Could you check a few things on this drawing? It's one solid part, dimensions in mm from its lowest x, y, z. A direction names the side the tool comes from. Round coordinates to 2 decimals unless told otherwise and drop trailing zeros. Order: outer loops, then holes, each group sorted by start corner. A loop starts at its lowest first (then second) coordinate and runs counter-clockwise, first axis right, second up. Notation, with made-up numbers: M -21,58.25 L 37,58.25 A22 cw 37,83.25 Z; hole C -2.75,-29.5 d9. An arc over 180 degrees is marked long. Answer as a JSON object with one key per item and string values. Group by question number.
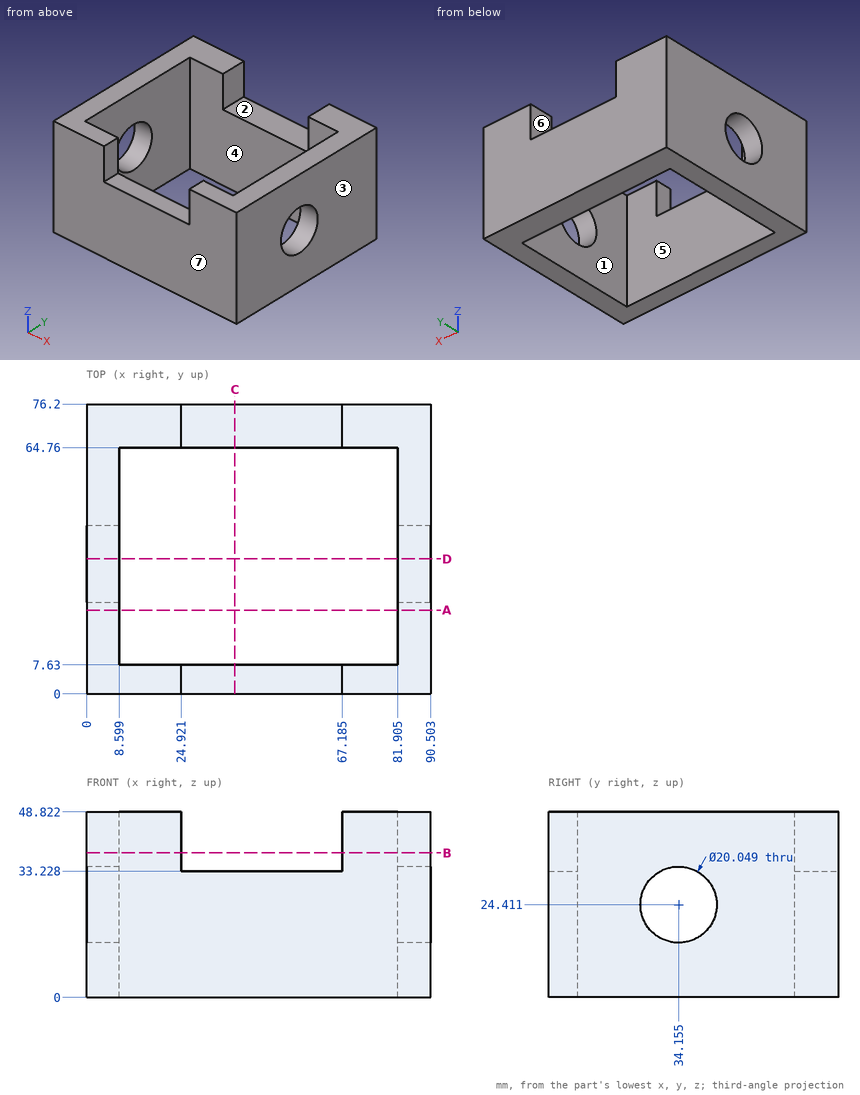
1) If we section it at B-B on z = 38: Write out the boundary of the cut face in (x, y) (1 decimal), plus the area to 3 significant figures.
2) If we section it at C-C on x = 39: Write out the boundary of the cut face in (y, z), plus the area to 3 significant figures.
3) If we section it at A-A on y = 22: Write out the boundary of the cut face in (x, z) (1 decimal).
4) Which directions (+Z, -Z, +X, -X, +Y, -Y) give clear straight access to the entire face, cutting with the end or side of a thin tool? Please do the marked faces 1, 2 and 3.
5) We'd pull the mould along Y, two halves only. Please class the marked faces 4, 5, 6 and 7: +Y half, -Y half, draft (parallel to the pull), parting line (faces both ways), or undercut.
6) If we section it at D-D on y = 35.5: Write out the boundary of the cut face in (x, z) (1 decimal).
7) For pin 1 (4 mm diameter, centred on x = 41.5, y = 5.5, fed in from +Z), with a flat end and sliding along its axis, tell me the tip position at first contact or that it passes through.
8) I need wall thicknesses on line 1 along Y through (x, z) = (38.5, 11); line 2 along X through (y, z) = (32, 35) (1 decimal); line 3 along Z through (x, y) = (44.5, 68). Which ranges of each line are inside material? Lowest first, please.
Findings:
{
 "1": {"outline": "M 0,0 L 24.9,0 L 24.9,7.6 L 8.6,7.6 L 8.6,64.8 L 24.9,64.8 L 24.9,76.2 L 0,76.2 Z; M 67.2,0 L 90.5,0 L 90.5,76.2 L 67.2,76.2 L 67.2,64.8 L 81.9,64.8 L 81.9,7.6 L 67.2,7.6 Z", "area": "1,900 mm^2"},
 "2": {"outline": "M 0,0 L 7.63,0 L 7.63,33.23 L 0,33.23 Z; M 64.76,0 L 76.2,0 L 76.2,33.23 L 64.76,33.23 Z", "area": "634 mm^2"},
 "3": {"outline": "M 0,0 L 8.6,0 L 8.6,48.8 L 0,48.8 Z; M 81.9,0 L 90.5,0 L 90.5,48.8 L 81.9,48.8 Z"},
 "4": {"face 1": "+Z, -Z", "face 2": "+Z, +Y, -Y", "face 3": "+Z, -Z, +X, +Y, -Y"},
 "5": {"face 4": "undercut", "face 5": "undercut", "face 6": "draft", "face 7": "-Y half"},
 "6": {"outline": "M 0,0 L 8.6,0 L 8.6,14.5 L 0,14.5 Z; M 0,34.3 L 8.6,34.3 L 8.6,48.8 L 0,48.8 Z; M 81.9,0 L 90.5,0 L 90.5,14.5 L 81.9,14.5 Z; M 81.9,34.3 L 90.5,34.3 L 90.5,48.8 L 81.9,48.8 Z"},
 "7": {"pin 1": "stops at z = 33.23"},
 "8": {"line 1": "y = 0 to 7.63, 64.76 to 76.2", "line 2": "x = 0 to 8.6, 81.9 to 90.5", "line 3": "z = 0 to 33.23"}
}
